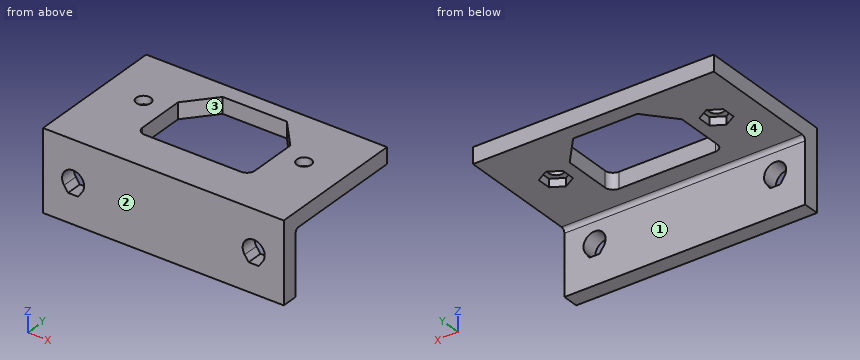
```python
from build123d import *

# Parameters (mm, degrees)
SALIENTE_EXTRUIR1_DEPTH = 30
CROQUIS2_R              = 1.8
CORTAR_EXTRUIR1_DEPTH   = 21
CORTAR_EXTRUIR2_DEPTH   = 36
REDONDEO1_R             = 1
CORTAR_EXTRUIR3_DEPTH   = 2


with BuildPart() as part:
    # Croquis1 → Saliente-Extruir1 (new body, symmetric)
    with BuildSketch(Plane(origin=(0, 0, 0), x_dir=(0, 0, -1), z_dir=(1, 0, 0))):
        Polygon((0, 0), (0, 35), (4, 35), (4, 4), (20, 4), (20, 0), align=None)
    extrude(amount=SALIENTE_EXTRUIR1_DEPTH, both=True)

    # Croquis2 → Cortar-Extruir1 (cut, through all)
    with BuildSketch(Plane.XY):
        with Locations((-20, 20.5)):
            Circle(CROQUIS2_R)
        with Locations((20, 20.5)):
            Circle(CROQUIS2_R)
        with BuildLine():
            Line((-12, 10), (12, 10))
            ThreePointArc((12, 10), (13.414213562, 10.585786438), (14, 12))
            Line((14, 12), (14, 24))
            Line((14, 24), (8, 31))
            Line((8, 31), (-8, 31))
            Line((-8, 31), (-14, 24))
            Line((-14, 24), (-14, 12))
            ThreePointArc((-14, 12), (-13.414213562, 10.585786438), (-12, 10))
        make_face()
    extrude(amount=-CORTAR_EXTRUIR1_DEPTH, mode=Mode.SUBTRACT)

    # Croquis3 → Cortar-Extruir2 (cut, through all)
    with BuildSketch(Plane.XZ):
        with BuildLine():
            Line((-24.747814832, -11.58424382), (-23.75, -13))
            Line((-23.75, -13), (-21.25, -13))
            Line((-21.25, -13), (-20.252185168, -11.58424382))
            ThreePointArc((-20.252185168, -11.58424382), (-22.5, -7.25), (-24.747814832, -11.58424382))
        make_face()
        with BuildLine():
            Line((20.252185168, -11.58424382), (21.25, -13))
            Line((21.25, -13), (23.75, -13))
            Line((23.75, -13), (24.747814832, -11.58424382))
            ThreePointArc((24.747814832, -11.58424382), (22.5, -7.25), (20.252185168, -11.58424382))
        make_face()
    extrude(amount=-CORTAR_EXTRUIR2_DEPTH, mode=Mode.SUBTRACT)

    # Redondeo1
    redondeo1_edges = [part.edges().sort_by_distance(p)[0] for p in [
        (0, 4, -4),
    ]]
    fillet(redondeo1_edges, radius=REDONDEO1_R)

    # Croquis4 → Cortar-Extruir3 (cut)
    with BuildSketch(Plane(origin=(0, 0, -4), x_dir=(-1, 0, 0), z_dir=(0, 0, -1))):
        Polygon((-17, 18.767949192), (-17, 22.232050808), (-20, 23.964101615), (-23, 22.232050808), (-23, 18.767949192), (-20, 17.035898385), align=None)
        Polygon((17, 18.767949192), (20, 17.035898385), (23, 18.767949192), (23, 22.232050808), (20, 23.964101615), (17, 22.232050808), align=None)
    extrude(amount=-CORTAR_EXTRUIR3_DEPTH, mode=Mode.SUBTRACT)


solid = part.part
```
Read the model definition and answer for the solid it produces. Units are mm, in the model's axes. Face numbers are marked on the shaded views. A direction names the side the tool comes from. Round coordinates to 2 decimals unless told otherwise and drop trailing zeros. Write each loop counter-clockwise with the first axis right and the second up, starting at its lowest first coordinate (ties: lowest second). Pieces come first, ordered by that corner, then holes. Notation, with made-up numbers: (25.25, -19.75) -> (44.25, -19.75) arc R16 ccw to (44.25, -2.75) -> close; hole circle Ø9 at (-28, -17.75). An arc over 180 degrees is marked (long way). Answer in a Markdown table with one row per item. Add a question column.
1) Consider line 1 (X direction, y = 2.4, z = -10); line 2 (Y direction, x = 20, z = -0.7); line 3 (Y direction, x = 1.5, z = -1.5). Determine where each line is inside the solid, lowest interval first.
2) Find section D-D, the plane y = 25. Determine the outline of the cut face in (x, z).
3) Given P1, Ø1.5, axis at x = 3.5, z = -16.5, coming from the +Y side; P2, Ø4.5, axis at x = 22.5, z = -10, coming from the -Y side; P3, Ø5, axis at x = -18.5, y = 21.5, coming from the -Z side, each flat-ended and moving along its own axis, determine where each tip first touches the part or whether it passes through.
4) Which of the six approach directions +Z, -Z, +X, -X, +Y, -Y give full straight-line access (tool end or side, diameter ignored) to the marked faces 1 and 2?
5) Find section A-A, the plane x = 3. Determine the outline of the cut face in (y, z).
6) Find section C-C, the plane z = -10. Determine the outline of the cut face in (x, y), and give its area (3 significant figures).
7) Determine the mould class of the marked faces 3 and 4 for opening direction X: pulls with the +X half, pulls with the -X half, needs draft (parallel to the pull), parting line crosses it, or undercut.
8) Find section B-B, the plane y = 20.5. Determine the outline of the cut face in (x, z).
Findings below:
| question | item | result |
|---|---|---|
| 1 | line 1 | -30 to -25.25, -19.75 to 19.75, 25.25 to 30 |
| 1 | line 2 | 0 to 18.7, 22.3 to 35 |
| 1 | line 3 | 0 to 10, 31 to 35 |
| 2 | outline | (-30, -4) -> (-13.14, -4) -> (-13.14, 0) -> (-30, 0) -> close; (13.14, -4) -> (30, -4) -> (30, 0) -> (13.14, 0) -> close |
| 3 | P1 | y = 4 |
| 3 | P2 | through |
| 3 | P3 | z = -4 |
| 4 | face 1 | -Z, +X, -X, +Y |
| 4 | face 2 | +Z, -Z, +X, -X, -Y |
| 5 | outline | (0, -20) -> (4, -20) -> (4, -5) arc R1 cw to (5, -4) -> (10, -4) -> (10, 0) -> (0, 0) -> close; (31, -4) -> (35, -4) -> (35, 0) -> (31, 0) -> close |
| 6 | outline | (-30, 0) -> (-25.25, 0) -> (-25.25, 4) -> (-30, 4) -> close; (-19.75, 0) -> (19.75, 0) -> (19.75, 4) -> (-19.75, 4) -> close; (25.25, 0) -> (30, 0) -> (30, 4) -> (25.25, 4) -> close |
| 6 | area | 196 mm² |
| 7 | face 3 | undercut |
| 7 | face 4 | needs draft |
| 8 | outline | (-30, -4) -> (-23, -4) -> (-23, -2) -> (-21.8, -2) -> (-21.8, 0) -> (-30, 0) -> close; (-18.2, -2) -> (-17, -2) -> (-17, -4) -> (-14, -4) -> (-14, 0) -> (-18.2, 0) -> close; (14, -4) -> (17, -4) -> (17, -2) -> (18.2, -2) -> (18.2, 0) -> (14, 0) -> close; (21.8, -2) -> (23, -2) -> (23, -4) -> (30, -4) -> (30, 0) -> (21.8, 0) -> close |
